from build123d import *

# Parameters (mm, degrees)
SKETCH1_W           = 28.8
SKETCH1_H           = 40
BOSS_EXTRUDE1_DEPTH = 3.1
SKETCH2_R           = 2.5
SKETCH2_W           = 3.1
SKETCH2_H           = 35
CUT_EXTRUDE1_DEPTH  = 4.1
SKETCH3_W           = 16.4
SKETCH3_H           = 42.5
SKETCH3_R           = 2.5
BOSS_EXTRUDE2_DEPTH = 3.1
FILLET1_R           = 7.5
BOSS_EXTRUDE3_DEPTH = 3.1


with BuildPart() as part:
    # Sketch1 → Boss-Extrude1 (new body)
    with BuildSketch(Plane.XY):
        Rectangle(SKETCH1_W, SKETCH1_H)
    extrude(amount=BOSS_EXTRUDE1_DEPTH)

    # Sketch2 → Cut-Extrude1 (cut, through all)
    with BuildSketch(Plane.XY.offset(3.1)):
        with Locations((0, -7.5)):
            Circle(SKETCH2_R)
        with Locations((-9.75, -2.5)):
            Rectangle(SKETCH2_W, SKETCH2_H)
        with Locations((9.75, -2.5)):
            Rectangle(SKETCH2_W, SKETCH2_H)
    extrude(amount=-CUT_EXTRUDE1_DEPTH, mode=Mode.SUBTRACT)

    # Sketch3 → Boss-Extrude2 (add, through all)
    with BuildSketch(Plane.XY.offset(3.1)):
        with Locations((0, -41.25)):
            Rectangle(SKETCH3_W, SKETCH3_H)
        with Locations((0, -57.5)):
            Circle(SKETCH3_R, mode=Mode.SUBTRACT)
    extrude(amount=-BOSS_EXTRUDE2_DEPTH)

    # Fillet1
    fillet1_edges = [part.edges().sort_by_distance(p)[0] for p in [
        (-8.2, -62.5, 1.55),
        (8.2, -62.5, 1.55),
    ]]
    fillet(fillet1_edges, radius=FILLET1_R)

    # Sketch4 → Boss-Extrude3 (add, through all)
    with BuildSketch(Plane(origin=(0, 0, 0), x_dir=(-1, 0, 0), z_dir=(0, 0, -1))):
        Polygon((-14.4, 20), (-14.4, -20), (-114.4, -12.5), (-114.4, -9.05), (-94.4, -9.05), (-94.4, -5.95), (-114.4, -5.95), (-114.4, -2.5), align=None)
    extrude(amount=-BOSS_EXTRUDE3_DEPTH)


solid = part.part
The listing builds one solid part. Answer for the finished solid, in the listing's coordinates (mm). A direction names the side the tool comes from. Round coordinates to 2 decimals unless told otherwise and drop trailing zeros. Loops run counter-clockwise (first coordinate to the right, second up) from the corner with the lowest first, then second, coordinate; pieces in that order, holes last. Notation, with made-up numbers: M 30,76 L 75,76 A20 cw 75,109 Z; hole C 52,-31 d10. An arc over 180 degrees is marked long. Write each question's results on one line, items separated by ' | '. Start each with the question number.
1) Each of these flat-tipped pins is pushed along its axis until it touches: pin 1 (6.5 mm diameter, centred on x = 0, y = -57.5, fed in from +Z); pin 2 (1.5 mm diameter, centred on x = 13, z = 1.5, fed in from -Y); pin 3 (1.6 mm diameter, centred on x = -10, z = 1.5, fed in from -Y). Where does it stop, or does it pass through?
2) Straight lines are drawn through the part: probe 1 along Y at (x, z) = (0, 1.35); probe 2 along X at (y, z) = (-12, 1.35); probe 3 along X at (y, z) = (-23.5, 2.6). For each, find the intervals that lie inside material, in ascending order.
3) Determine the mould class of faces 1 (the flat face through (-11.3, -3, 2)), 2 (the flat face through (-14.4, 0, 2)), 3 (the cylindrical face through (1.34, -55.39, 1.57)), 4 (the flat face through (35, -12, 0)) for opening direction X: pulls with the +X half, pulls with the -X half, needs draft (parallel to the pull), parting line crosses it, or undercut.
4) Find section C-C on y = -57.5. Write down the section's boundary in (x, z), plus the area to 3 significant figures.
5) Find section A-A on y = -7.5. Write down the section's boundary in (x, z).
6) Find section D-D on x = 16. Write down the section's boundary in (y, z), plus the area to 3 significant figures.
7) Find section B-B on z = 1.2. Write down the section's boundary in (x, y).
8) Which of the six approach directions +Z, -Z, +X, -X, +Y, -Y give full straight-line access (tool end or side, diameter ignored) to faces 5 (the flat face through (-10, 15, 2)), 6 (the flat face through (-13, -20, 2)), 7 (the flat face through (104, -5.95, 2))?
Final values:
1) pin 1: z = 3.1 | pin 2: y = -20 | pin 3: y = 15
2) probe 1: -62.5 to -60, -55 to -10, -5 to 20 | probe 2: -14.4 to -11.3, -8.2 to 8.2, 11.3 to 114.4 | probe 3: -8.2 to 8.2
3) face 1: undercut | face 2: pulls with the -X half | face 3: undercut | face 4: needs draft
4) outline: M -7.77,0 L -2.5,0 L -2.5,3.1 L -7.77,3.1 Z; M 2.5,0 L 7.77,0 L 7.77,3.1 L 2.5,3.1 Z | area: 32.7 mm²
5) outline: M -14.4,0 L -11.3,0 L -11.3,3.1 L -14.4,3.1 Z; M -8.2,0 L -2.5,0 L -2.5,3.1 L -8.2,3.1 Z; M 2.5,0 L 8.2,0 L 8.2,3.1 L 2.5,3.1 Z; M 11.3,0 L 94.4,0 L 94.4,3.1 L 11.3,3.1 Z
6) outline: M -19.88,0 L 19.64,0 L 19.64,3.1 L -19.88,3.1 Z | area: 123 mm²
7) outline: M -14.4,-20 L -11.3,-20 L -11.3,15 L -8.2,15 L -8.2,-55 A7.5 ccw -0.7,-62.5 L 0.7,-62.5 A7.5 ccw 8.2,-55 L 8.2,15 L 11.3,15 L 11.3,-20 L 14.4,-20 L 114.4,-12.5 L 114.4,-9.05 L 94.4,-9.05 L 94.4,-5.95 L 114.4,-5.95 L 114.4,-2.5 L 14.4,20 L -14.4,20 Z; hole C 0,-57.5 d5; hole C 0,-7.5 d5
8) face 5: +Z, -Z, -Y | face 6: +Z, -Z, -X, -Y | face 7: +Z, -Z, +X
